from build123d import *

# Parameters (mm, degrees)
SKETCH1_R      = 56
EXTRUDE1_DEPTH = 38
EXTRUDE2_DEPTH = 28
SKETCH3_R      = 34.5
EXTRUDE3_DEPTH = 256.234206172


with BuildPart() as part:
    # Sketch1 → Extrude1 (new body)
    with BuildSketch(Plane.XY):
        with BuildLine():
            Line((-105, -40), (-90.012499132, -40))
            ThreePointArc((-90.012499132, -40), (0, -98.5), (90.012499132, -40))
            Line((90.012499132, -40), (105, -40))
            Line((105, -40), (105, 40))
            Line((105, 40), (90.012499132, 40))
            ThreePointArc((90.012499132, 40), (0, 98.5), (-90.012499132, 40))
            Line((-90.012499132, 40), (-105, 40))
            Line((-105, 40), (-105, -40))
        make_face()
        Circle(SKETCH1_R, mode=Mode.SUBTRACT)
    extrude(amount=EXTRUDE1_DEPTH)

    # Sketch2 → Extrude2 (add)
    with BuildSketch(Plane.ZY.offset(105)):
        with BuildLine():
            Line((0, 40), (-22.561596833, 40))
            ThreePointArc((-22.561596833, 40), (-106.5, 0), (-22.561596833, -40))
            Line((-22.561596833, -40), (0, -40))
            Line((0, -40), (0, 40))
        make_face()
    extrude2 = extrude(amount=-EXTRUDE2_DEPTH)

    # Mirror1: Extrude2 across plane
    add(extrude2.mirror(Plane(origin=(0, 0, 0), x_dir=(0, 0, 1), z_dir=(1, 0, 0))))

    # Sketch3 → Extrude3 (cut, through all)
    with BuildSketch(Plane.ZY.offset(105)):
        with Locations((-55, 0)):
            Circle(SKETCH3_R)
    extrude(amount=-EXTRUDE3_DEPTH, mode=Mode.SUBTRACT)


solid = part.part
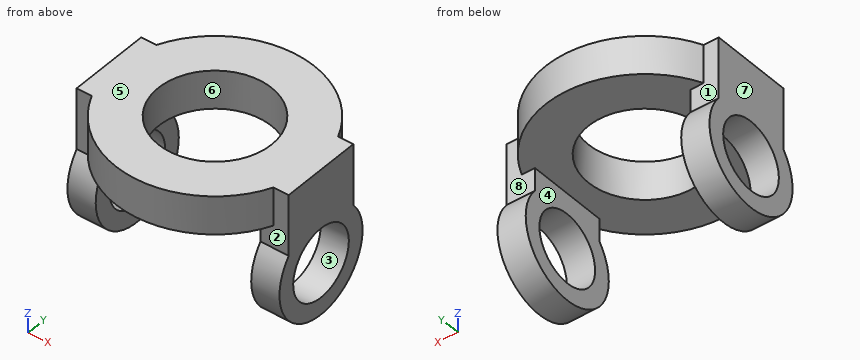
Here's how the part is built. I have some questions about the finished solid (model axes, mm). Face numbers are marked on the shaded views. A direction names the side the tool comes from. Round coordinates to 2 decimals unless told otherwise and drop trailing zeros. Loops run counter-clockwise (first coordinate to the right, second up) from the corner with the lowest first, then second, coordinate; pieces in that order, holes last.
1. If we section it at A-A on z = -55: Write out the boundary of the cut face in (x, y).
Answer list:
outline: (-105, -51.5) - (-77, -51.5) - (-77, -34.5) - (-105, -34.5) - close; (-105, 34.5) - (-77, 34.5) - (-77, 51.5) - (-105, 51.5) - close; (77, -51.5) - (105, -51.5) - (105, -34.5) - (77, -34.5) - close; (77, 34.5) - (105, 34.5) - (105, 51.5) - (77, 51.5) - close
2. If we section it at D-D on z = -6: Write out the boundary of the cut face in (x, y).
Answer list:
outline: (-105, -40) - (-77, -40) - (-77, 40) - (-105, 40) - close; (77, -40) - (105, -40) - (105, 40) - (77, 40) - close
3. Which directions (+Z, -Z, +X, -X, +Y, -Y) give clear straight access to the entire face, cutting with the end or side of a thin tool? Please do the marked faces 1, 2, 3, 4 and 5.
Answer list:
face 1: -X, +Y
face 2: +X, -Y
face 3: +X, -X
face 4: -Z, +Y, -Y
face 5: +Z, +X, -X, +Y, -Y
4. If we section it at B-B on x = 0: Write out the boundary of the cut face in (y, z).
Answer list:
outline: (-98.5, 0) - (-56, 0) - (-56, 38) - (-98.5, 38) - close; (56, 0) - (98.5, 0) - (98.5, 38) - (56, 38) - close
5. We'd pull the mould along Y, two halves only. Please class the marked faces 6, 7 and 8: +Y half, -Y half, draft (parallel to the pull), parting line (faces both ways), or undercut.
Answer list:
face 6: undercut
face 7: draft
face 8: +Y half
6. If we section it at C-C on y = 0: Write out the boundary of the cut face in (x, z).
Answer list:
outline: (-105, -106.5) - (-77, -106.5) - (-77, -89.5) - (-105, -89.5) - close; (-105, -20.5) - (-77, -20.5) - (-77, 0) - (-56, 0) - (-56, 38) - (-105, 38) - close; (56, 0) - (77, 0) - (77, -20.5) - (105, -20.5) - (105, 38) - (56, 38) - close; (77, -106.5) - (105, -106.5) - (105, -89.5) - (77, -89.5) - close
7. If I drill on line 1 along X through (y, z) = (30.5, -38.5); line 2 along Y through (x, z) = (-89, -55); line 3 along Z through (x, y) = (69.5, -24.5), over which ranges is the centre line in solid material (lowest first)?
Answer list:
line 1: x = -105 to -77, 77 to 105
line 2: y = -51.5 to -34.5, 34.5 to 51.5
line 3: z = 0 to 38
8. For P1, Ø8, axis at x = 76, z = -79.5, coming from the +Y side; P2, Ø1.5, axis at x = -13, y = -71, coming from the -Z side; P3, Ø14, axis at x = -97, z = -7, coming from the -Y side, each with a flat end and sliding along its axis, tell me the tip position at first contact or that it passes through.
Answer list:
P1: stops at y = 47.19
P2: stops at z = 0
P3: stops at y = -40
